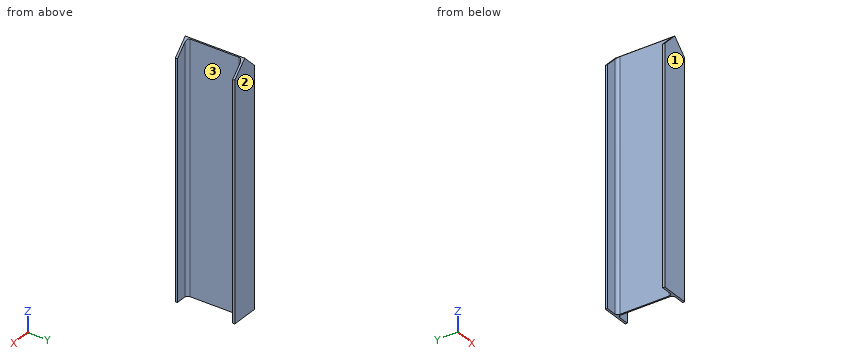
Autodesk Inventor part; units mm, degrees
ref_plane "Start Plane" through (0, 0, 0) normal (0, 0, 1) x (1, 0, 0)
ref_plane "End Plane" through (0, 0, 1500) normal (0, 0, 1) x (1, 0, 0)
ref_plane "Work Plane4" through (85, 0, 1585) normal (-0.7071, 0, 0.7071) x (0.7071, 0, 0.7071)
ref_plane "Start Plane" through (0, 0, 0) normal (0, 0, 1) x (1, 0, 0)
ref_plane "End Plane" through (0, 0, 1500) normal (0, 0, 1) x (1, 0, 0)
sketch "Sketch" plane through (0, 0, 0) normal (0, 0, 1) x (1, 0, 0)
  line L0 (-85, 167.3) -> (-22, 167.3)
  line L1 (-85, 180) -> (-85, 167.3)
  line L2 (85, 180) -> (-85, 180)
  line L3 (85, 167.3) -> (85, 180)
  line L4 (22, 167.3) -> (85, 167.3)
  line L5 (4, -149.3) -> (4, 149.3)
  line L6 (85, -167.3) -> (22, -167.3)
  line L7 (85, -180) -> (85, -167.3)
  line L8 (-85, -167.3) -> (-85, -180)
  line L9 (-22, -167.3) -> (-85, -167.3)
  line L10 (-4, 149.3) -> (-4, -149.3)
  line L11 (0, -252) -> (0, 252) construction
  line L12 (-4, -167.3) -> (4, -167.3) construction
  arc A0 (-22, -167.3) -> (-4, -149.3) centre (-22, -149.3) ccw
  arc A1 (-4, 149.3) -> (-22, 167.3) centre (-22, 149.3) ccw
  arc A2 (22, 167.3) -> (4, 149.3) centre (22, 149.3) ccw
  arc A3 (4, -149.3) -> (22, -167.3) centre (22, -149.3) ccw
  line L13 (-119, 0) -> (119, 0) construction
  line L14 (-85, -180) -> (85, -180)
  point P0 (-4, 167.3)
  point P1 (4, 167.3)
  point P2 (0, 0)
  point P3 (0, -167.3)
  point P4 (0, 0)
  dimension "d1" = 360
  dimension "d3" = 12.7
  dimension "d5" = 8
  dimension "d7" = 170
  dimension "d13" = 18
  dimension "d14" = 180
  dimension "d15" = 85
extrude "Body" add sketch "Sketch" along normal up to surface (1500 mm away) from surface at 0
sketch "Sketch3" plane through (0, 0, 0) normal (0, 0, 1) x (1, 0, 0)
  line L0 (0, 0) -> (10, 0)
ref_plane "Work Plane3" through (0, 0, 0) normal (0, -1, 0) x (1, 0, 0)
ref_plane "Work Plane4" through (85, 0, 1585) normal (-0.7071, 0, 0.7071) x (0.7071, 0, 0.7071)
split "Split1" plane through (85, 0, 1585) removes the side toward (-0.7071, 0, 0.7071)
ref_plane "Work Plane5" through (-85, 0, 1585) normal (0.7071, 0, 0.7071) x (0.7071, 0, -0.7071)
split "Split2" plane through (-85, 0, 1585) removes the side toward (0.7071, 0, 0.7071)
sketch "Sketch4" plane through (0, 0, 0) normal (0, -1, 0) x (1, 0, 0)
  line L0 (-2, 0) -> (12, 0)
  line L1 (-2, 1500) -> (12, 1500)
  dimension "d19" = 1500
equation "\"d1\" = ParH"
equation "\"d3\" = t2"
equation "\"d7\" = b"
equation "\"d13\" = R1"
equation "\"d14\" = 0.5 * d1"
equation "\"d15\" = 0.5 * d7"
equation "\"d8\" = G_L"
equation "\"b\" = 170"
equation "\"ParH\" = 360"
equation "\"R1\" = 18"
equation "\"G_L\" = d19"
equation "\"t1\" = 8"
equation "\"t2\" = 12.7"
equation "\"G_OFFSET_START\" = 0"
equation "\"G_OFFSET_END\" = 0"
properties part number "DIN 1025 - IPE 360-1500" material "Steel, Mild"
Input: part model. Units: mm. Frame: model coordinates. Face numbers are marked on the shaded views. Give positions to 0.01 mm unless a question says otherwise; leave off trailing zeros. Order: outer loops, then holes, each group sorted by start corner. A loop starts at its lowest first (then second) coordinate and runs counter-clockwise, first axis right, second up. Notation, with made-up numbers: M 26.5,1.5 L 62.5,1.5 A27 ccw 62.5,38.5 Z; hole C 30.25,78.25 d7. An arc over 180 degrees is marked long. One line per question, with ' | ' between items.
1) Section D-D on x = 39. Output: boundary loops of the cut face in (y, z).
Filled in:
outline: M -180,0 L -167.3,0 L -167.3,1461 L -180,1461 Z; M 167.3,0 L 180,0 L 180,1461 L 167.3,1461 Z
2) Section A-A on x = -46.5. Output: boundary loops of the cut face in (y, z).
Filled in:
outline: M -180,0 L -167.3,0 L -167.3,1453.5 L -180,1453.5 Z; M 167.3,0 L 180,0 L 180,1453.5 L 167.3,1453.5 Z
3) Section B-B on z = 1259. Output: boundary loops of the cut face in (x, y).
Filled in:
outline: M -85,-180 L 85,-180 L 85,-167.3 L 22,-167.3 A18 cw 4,-149.3 L 4,149.3 A18 cw 22,167.3 L 85,167.3 L 85,180 L -85,180 L -85,167.3 L -22,167.3 A18 cw -4,149.3 L -4,-149.3 A18 cw -22,-167.3 L -85,-167.3 Z
4) Draft query along Y for the marked faces 1, 2 and 3. Return one class per face: pulls with the +Y half, pulls with the -Y half, needs draft (parallel to the pull), parting line crosses it, or undercut.
Filled in:
face 1: pulls with the -Y half | face 2: pulls with the +Y half | face 3: undercut
5) Contact query for flat-ended pins moving along their axis: P1, Ø5, axis at y = -39, z = 282.5, coming from the -X side; P2, Ø6, axis at y = -40, z = 866.5, coming from the +X side. Output: stop coordinate, or through.
Filled in:
P1: stops at x = -4 | P2: stops at x = 4
6) Section C-C on y = -66.5. Output: boundary loops of the cut face in (x, z).
Filled in:
outline: M -4,0 L 4,0 L 4,1496 L 0,1500 L -4,1496 Z
7) Ray query, L1, parallel to Y at x = 29.5, z = 1043.5; L2, parallel to Y at x = 20, z = 321.5; L3, parallel to X at y = -33, z = 423. Return the intervals inside material, ascending.
Filled in:
L1: y = -180 to -167.3, 167.3 to 180 | L2: y = -180 to -167.19, 167.19 to 180 | L3: x = -4 to 4
